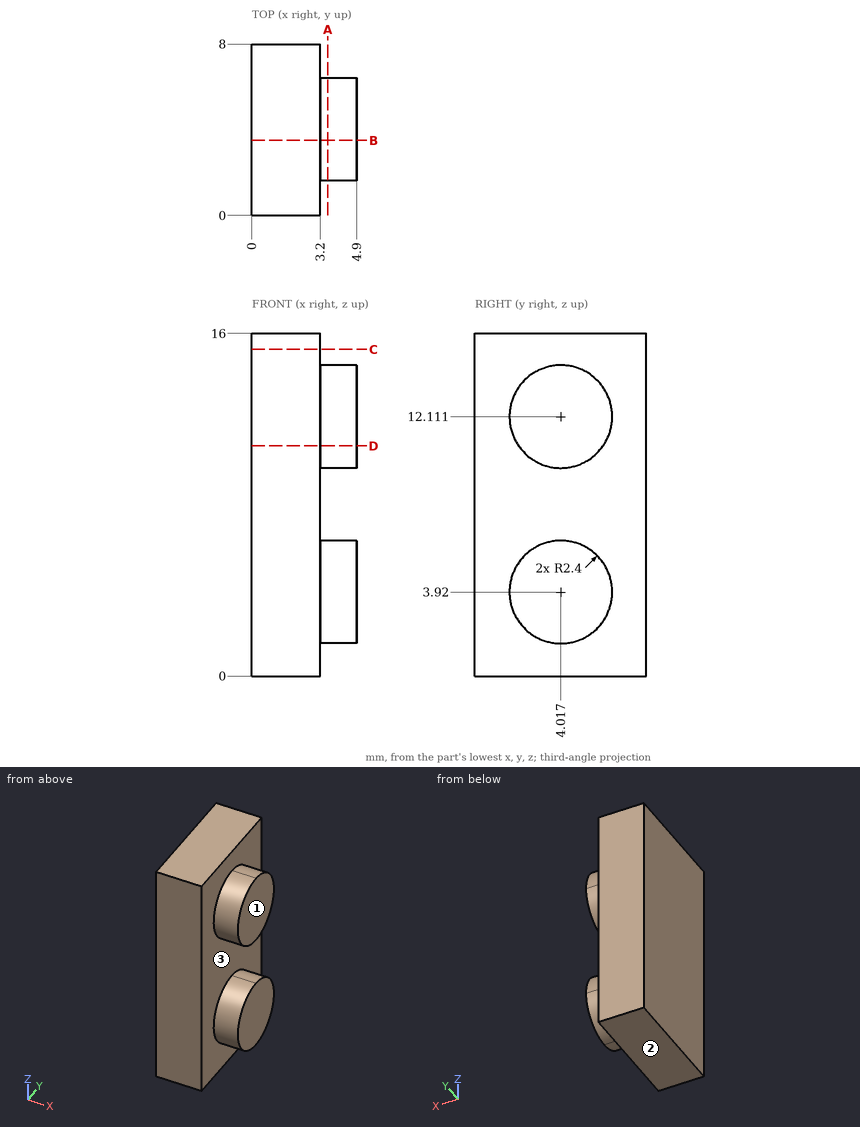
Drawing for the job (mm, zero at the part's lowest x, y, z). Round coordinates to 2 decimals unless told otherwise and drop trailing zeros. Order: outer loops, then holes, each group sorted by start corner. A loop starts at its lowest first (then second) coordinate and runs counter-clockwise, first axis right, second up.
Item 1: Saw through at A-A on x = 3.55. Write the cut outline in (y, z).
Item 2: Saw through at B-B on y = 3.5. Write the cut outline in (x, z) (1 decimal).
Item 3: Mould opens along Z. For the marked faces 1, 2 and 3 say: pulls with the +Z half, pulls with the -Z half, needs draft (parallel to the pull), parting line crosses it, or undercut.
Item 4: Probe line 1 along X through (y, z) = (2.25, 14.25); line 2 along Z through (x, y) = (4.1, 3.5) (1 decimal); line 3 along Z through (x, y) = (3.75, 5). List the from-to ranges inside material, lowest first.
Item 5: Saw through at D-D on z = 10.75. Write the cut outline in (x, y), then the cut area to 3 significant figures.
Item 6: Saw through at C-C on z = 15.25. Write the cut outline in (x, y), then the cut area to 3 significant figures.
Reported:
1. outline: circle Ø4.8 at (4.02, 3.92); circle Ø4.8 at (4.02, 12.11)
2. outline: (0, 0) - (3.2, 0) - (3.2, 1.6) - (4.9, 1.6) - (4.9, 6.3) - (3.2, 6.3) - (3.2, 9.8) - (4.9, 9.8) - (4.9, 14.5) - (3.2, 14.5) - (3.2, 16) - (0, 16) - close
3. face 1: needs draft
3. face 2: pulls with the -Z half
3. face 3: undercut
4. line 1: x = 0 to 3.2
4. line 2: z = 1.6 to 6.3, 9.8 to 14.5
4. line 3: z = 1.73 to 6.11, 9.92 to 14.3
5. outline: (0, 0) - (3.2, 0) - (3.2, 2.04) - (4.9, 2.04) - (4.9, 5.99) - (3.2, 5.99) - (3.2, 8) - (0, 8) - close
5. area: 32.3 mm2
6. outline: (0, 0) - (3.2, 0) - (3.2, 8) - (0, 8) - close
6. area: 25.6 mm2
